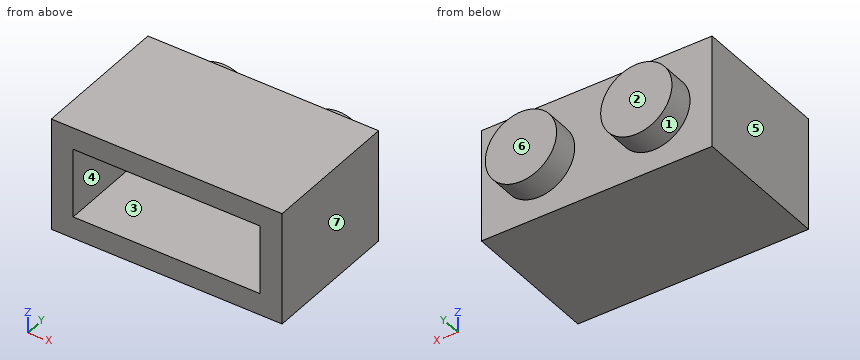
```python
from build123d import *

# Parameters (mm, degrees)
SKETCH1_W           = 15.85
SKETCH1_H           = 7.75
BOSS_EXTRUDE1_DEPTH = 9.6
SKETCH2_R           = 2.45
BOSS_EXTRUDE2_DEPTH = 1.8
SHELL1_T            = -1.5


with BuildPart() as part:
    # Sketch1 → Boss-Extrude1 (new body)
    with BuildSketch(Plane(origin=(0, 0, 0), x_dir=(1, 0, 0), z_dir=(0, 1, 0))):
        Rectangle(SKETCH1_W, SKETCH1_H)
    extrude(amount=-BOSS_EXTRUDE1_DEPTH)

    # Sketch2 → Boss-Extrude2 (add)
    with BuildSketch(Plane(origin=(0, 0, 0), x_dir=(1, 0, 0), z_dir=(0, 1, 0))):
        with Locations(Location((-3.9625, 0, 0), (0, 0, 270))):
            Circle(SKETCH2_R)
        with Locations(Location((3.9625, 0, 0), (0, 0, 90))):
            Circle(SKETCH2_R)
    extrude(amount=BOSS_EXTRUDE2_DEPTH)

    # Shell1
    shell1_openings = [part.faces().sort_by_distance(p)[0] for p in [
        (0, -9.6, 0),
    ]]
    offset(amount=SHELL1_T, openings=shell1_openings, kind=Kind.INTERSECTION)


solid = part.part
```
CAD build for the part. Positions are in the model's coordinates, mm. Face numbers are marked on the shaded views. A direction names the side the tool comes from. Coordinates: 2 decimals unless noted, no trailing zeros. Loops run counter-clockwise (first coordinate to the right, second up) from the corner with the lowest first, then second, coordinate; pieces in that order, holes last. Notation, with made-up numbers: (-25, -6) - (-3, -6) arc R10 cw to (-3, 3) - close; hole circle Ø4 at (50, -8). An arc over 180 degrees is marked (long way). Use CSV: the item, a comma, the result in double quotes. Start each with the question number.
Q1. Probe probe 1 along X at (y, z) = (-0.15, 0) (1 decimal); probe 2 along X at (y, z) = (-6.75, 1.25) (3 decimals); probe 3 along Z at (x, y) = (-3.75, -6) (3 decimals). List the from-to ranges inside material, lowest first. Write a range as from..to.
Q2. 3-axis set-ups, long thin cutter, end or side, ignore diameter. For the marked faces 1, 2 and 3: which of +Z, -Z, +X, -X, +Y, -Y reach the whole face in a straight line?
Q3. Cut at A-A, the plane y = -7.75. List the corners of the cut face in (x, z) (3 decimals).
Q4. Two-plate mould, pull along X, no slides. Class the marked faces 4, 5, 6 and 7: +X half, -X half, draft (parallel to the pull), parting line (faces both ways), or undercut.
Q5. Cut at B-B, the plane x = -0.5. List the corners of the cut face in (y, z) (3 decimals).
Q6. Drop flat-ended pins along their axis: P1, Ø1.4, axis at x = -2.5, z = 0, coming from the -Y side; P2, Ø2, axis at x = 0, z = 0.5, coming from the +Y side; P3, Ø0.6, axis at x = 4, z = 0, coming from the -Y side. Give the stop position or say it passes through.
Q7. Cut at C-C, the plane z = 0. List the corners of the cut face in (x, y) (1 decimal), then the cut area to 3 significant figures.
Q8. Cut at D-D, the plane z = -2. List the corners of the cut face in (x, y) (3 decimals), then the cut area to 3 significant figures.
Here are the results:
1,probe 1,"-7.9..-4.9, -3..3, 4.9..7.9"
1,probe 2,"-7.925..-6.425, 6.425..7.925"
1,probe 3,"-3.875..-2.375, 2.375..3.875"
2,face 1,"+Y"
2,face 2,"+Z, -Z, +X, -X, +Y"
2,face 3,"-Y"
3,outline,"(-7.925, -3.875) - (7.925, -3.875) - (7.925, 3.875) - (-7.925, 3.875) - close; hole (-6.425, -2.375) - (6.425, -2.375) - (6.425, 2.375) - (-6.425, 2.375) - close"
4,face 4,"undercut"
4,face 5,"-X half"
4,face 6,"draft"
4,face 7,"+X half"
5,outline,"(-9.6, -3.875) - (0, -3.875) - (0, 3.875) - (-9.6, 3.875) - (-9.6, 2.375) - (-1.5, 2.375) - (-1.5, -2.375) - (-9.6, -2.375) - close"
6,P1,"y = -1.5"
6,P2,"y = 0"
6,P3,"y = 0.3"
7,outline,"(-7.9, -9.6) - (-6.4, -9.6) - (-6.4, -1.5) - (-4.9, -1.5) - (-4.9, 0.3) - (-3, 0.3) - (-3, -1.5) - (3, -1.5) - (3, 0.3) - (4.9, 0.3) - (4.9, -1.5) - (6.4, -1.5) - (6.4, -9.6) - (7.9, -9.6) - (7.9, 0) - (6.4, 0) - (6.4, 1.8) - (1.5, 1.8) - (1.5, 0) - (-1.5, 0) - (-1.5, 1.8) - (-6.4, 1.8) - (-6.4, 0) - (-7.9, 0) - close"
7,area,"58.9 mm2"
8,outline,"(-7.925, -9.6) - (-6.425, -9.6) - (-6.425, -1.5) - (6.425, -1.5) - (6.425, -9.6) - (7.925, -9.6) - (7.925, 0) - (5.378, 0) - (5.378, 1.8) - (2.547, 1.8) - (2.547, 0) - (-2.547, 0) - (-2.547, 1.8) - (-5.378, 1.8) - (-5.378, 0) - (-7.925, 0) - close"
8,area,"58.3 mm2"
